```python
from build123d import *

# Parameters (mm, degrees)
SKETCH1_R           = 25.4
BOSS_EXTRUDE1_DEPTH = 33.274
SKETCH2_R           = 22.225
BOSS_EXTRUDE2_DEPTH = 19.05
SKETCH3_R           = 12.7
CUT_EXTRUDE2_DEPTH  = 64.467479673
BOSS_EXTRUDE3_DEPTH = 25.4
FILLET1_R           = 6.35
FILLET2_R           = 6.35
CUT_EXTRUDE3_DEPTH  = 154.088688922
BOSS_EXTRUDE4_DEPTH = 8.128
FILLET3_R           = 6.35


with BuildPart() as part:
    # Sketch1 → Boss-Extrude1 (new body)
    with BuildSketch(Plane.XY):
        Circle(SKETCH1_R)
    extrude(amount=BOSS_EXTRUDE1_DEPTH)

    # Sketch2 → Boss-Extrude2 (add)
    with BuildSketch(Plane.XY.offset(33.274)):
        with Locations(Location((0, 0, 0), (0, 0, 180))):
            Circle(SKETCH2_R)
    extrude(amount=BOSS_EXTRUDE2_DEPTH)

    # Sketch3 → Cut-Extrude2 (cut, through all)
    with BuildSketch(Plane.XY):
        Circle(SKETCH3_R)
    extrude(amount=CUT_EXTRUDE2_DEPTH, mode=Mode.SUBTRACT)

    # Sketch5 → Boss-Extrude3 (add)
    with BuildSketch(Plane(origin=(0, 0, 3.048), x_dir=(-1, 0, 0), z_dir=(0, 0, -1))):
        with BuildLine():
            Line((100.803124952, 12.7), (21.997045256, 12.7))
            ThreePointArc((21.997045256, 12.7), (24.534515988, 6.574003746), (25.4, 0))
            ThreePointArc((25.4, 0), (24.534515988, -6.574003746), (21.997045256, -12.7))
            Line((21.997045256, -12.7), (100.803124952, -12.7))
            ThreePointArc((100.803124952, -12.7), (100.053333913, -17.660418251), (99.059597973, -22.577777778))
            ThreePointArc((99.059597973, -22.577777778), (108.619825498, -37.782449747), (123.824497467, -28.222222222))
            ThreePointArc((123.824497467, -28.222222222), (125.578613792, 18.9476056), (109.985226281, 63.5))
            ThreePointArc((109.985226281, 63.5), (92.636703653, 68.148522628), (87.988181024, 50.8))
            ThreePointArc((87.988181024, 50.8), (96.298711326, 32.390094118), (100.803124952, 12.7))
        make_face()
    extrude(amount=-BOSS_EXTRUDE3_DEPTH)

    # Fillet1
    fillet1_edges = [part.edges().sort_by_distance(p)[0] for p in [
        (-100.803124952, 12.7, 15.748),
    ]]
    fillet(fillet1_edges, radius=FILLET1_R)

    # Fillet2
    fillet2_edges = [part.edges().sort_by_distance(p)[0] for p in [
        (-100.803124952, -12.7, 15.748),
    ]]
    fillet(fillet2_edges, radius=FILLET2_R)

    # Sketch6 → Cut-Extrude3 (cut, through all)
    with BuildSketch(Plane(origin=(0, 0, 3.048), x_dir=(-1, 0, 0), z_dir=(0, 0, -1))):
        with BuildLine():
            Line((44.45, -5.588), (82.55, -5.588))
            ThreePointArc((82.55, -5.588), (88.138, 0), (82.55, 5.588))
            Line((82.55, 5.588), (44.45, 5.588))
            ThreePointArc((44.45, 5.588), (38.862, 0), (44.45, -5.588))
        make_face()
        with BuildLine():
            ThreePointArc((117.620316517, -26.867892407), (119.3040242, 17.971430377), (104.485964967, 60.325))
            ThreePointArc((104.485964967, 60.325), (95.811703653, 62.649261314), (93.487442339, 53.975))
            ThreePointArc((93.487442339, 53.975), (106.745705863, 16.079700863), (105.239230568, -24.039693207))
            ThreePointArc((105.239230568, -24.039693207), (110.015673942, -31.644335781), (117.620316517, -26.867892407))
        make_face()
    extrude(amount=-CUT_EXTRUDE3_DEPTH, mode=Mode.SUBTRACT)

    # Sketch7 → Boss-Extrude4 (add)
    with BuildSketch(Plane.XY.offset(8.128)):
        with BuildLine():
            Line((-93.3255592, 12.7), (-21.997045256, 12.7))
            ThreePointArc((-21.997045256, 12.7), (-10.533208363, 23.11301628), (4.846548483, 24.93333046))
            Line((4.846548483, 24.93333046), (-91.719825153, 43.703932019))
            ThreePointArc((-91.719825153, 43.703932019), (-96.345611399, 32.250320373), (-99.547263147, 20.32))
            ThreePointArc((-99.547263147, 20.32), (-98.24424805, 15.033907372), (-93.3255592, 12.7))
        make_face()
    extrude(amount=BOSS_EXTRUDE4_DEPTH)

    # Fillet3
    # the kernel refuses this fillet: 6.35 mm, written as the material it adds along each edge
    with BuildSketch(Plane(origin=(-91.719825153, 43.703932019, 8.128), x_dir=(0.4664648604868203, 0.8845397299901295, 0), z_dir=(0, 0, 1))) as fillet3_piece_1:
        with BuildLine():
            CenterArc((8.551066202, -6.349980485), FILLET3_R, 90.142046539, 106.663020028)
            Line((2.472249714, -8.185869942), (1.864368065, -8.369458888))
            Line((1.864368065, -8.369458888), (-0.607881649, -0.183588946))
            Line((-0.607881649, -0.183588946), (-0.02578882, 0.634476112))
            ThreePointArc((-0.02578882, 0.634476112), (8.041755062, 0.643812976), (8.533749149, 0.634998049))
            Line((8.533749149, 0.634998049), (8.535323427, 0))
        make_face()
    extrude(amount=8.128)


solid = part.part
```
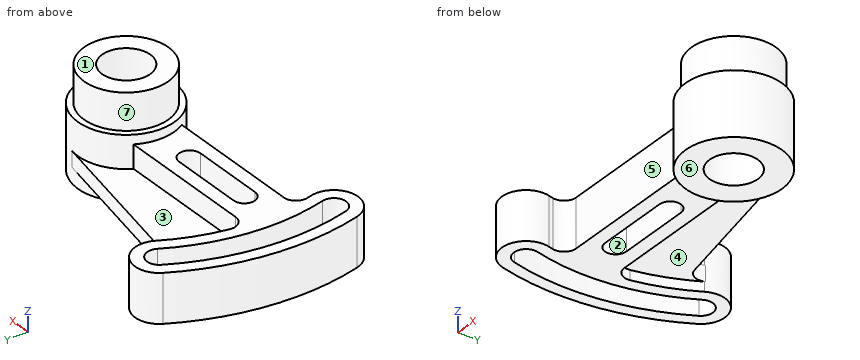
The model under review builds one solid part; all positions refer to its coordinate system, in mm. Face numbers are marked on the shaded views. A direction names the side the tool comes from. Give positions to 0.01 mm unless a question says otherwise; leave off trailing zeros. Order: outer loops, then holes, each group sorted by start corner. A loop starts at its lowest first (then second) coordinate and runs counter-clockwise, first axis right, second up. Notation, with made-up numbers: (-8.75, 4.25) - (25.25, 4.25) arc R22 ccw to (25.25, 28.25) - close; hole circle Ø1 at (77, 3). An arc over 180 degrees is marked (long way). Use CSV: the item, a comma, the result in double quotes. Start each with the question number.
Q1. We need section A-A, the plane y = 0. Write out the cut boundary in (x, z) (3 decimals), and give its area (3 significant figures).
Q2. To check wall thickness, follow line 1 along Y through (x, z) = (0, 26.5); line 2 along X through (y, z) = (0, 26); line 3 along Y through (x, z) = (0, 40.5) (3 decimals). State the ranges of each line that lie inside material, in increasing order. Write a range as [from, to].
Q3. We need section D-D, the plane z = 5. State how many separate pieces and enclosed holes the cut face has, and give its area (3 significant figures).
Q4. Clearance check with flat-ended pins moving along their axes: pin 1 Ø1 at (y, z) = (26.5, 12.5) entering from -X; pin 2 Ø1 at (x, z) = (-86, 24.5) entering from -Y; pin 3 Ø1.5 at (x, z) = (-47, 5) entering from +Y. State where each tip first meets the part, or that it passes through.
Q5. The part is to be moulded in two halves that separate along Y. For the marked faces 4, 5, 6 and 7, say which applies: +Y half, -Y half, draft (parallel to the pull), parting line (faces both ways), or undercut.
Q6. We need section B-B, the plane x = -73.5. Write out the cut boundary in (y, z), and give its area (3 significant figures).
Q7. We need section C-C, the plane y = 57.15. Write out the cut boundary in (x, z), and give its area (3 significant figures).
Q8. Tool access review of the marked faces 1, 2 and 3: name each direction out of +Z, -Z, +X, -X, +Y, -Y from which nothing blocks a thin tool from reaching the whole face with its end or side.
Outcome:
1,outline,"(-127, 3.048) - (-120.65, 3.048) - (-120.65, 28.448) - (-127, 28.448) - close; (-107.95, 3.048) - (-88.138, 3.048) - (-88.138, 28.448) - (-107.95, 28.448) - close; (-38.862, 3.048) - (-25.4, 3.048) - (-25.4, 0) - (-12.7, 0) - (-12.7, 52.324) - (-22.225, 52.324) - (-22.225, 33.274) - (-25.4, 33.274) - (-25.4, 28.448) - (-38.862, 28.448) - close; (12.7, 0) - (25.4, 0) - (25.4, 33.274) - (22.225, 33.274) - (22.225, 52.324) - (12.7, 52.324) - close"
1,area,"2,210 mm^2"
2,line 1,"y = [-25.4, -12.7], [12.7, 25.4]"
2,line 2,"x = [-127, -120.65], [-107.95, -88.14], [-38.86, -12.7], [12.7, 25.4]"
2,line 3,"y = [-22.225, -12.7], [12.7, 22.225]"
3,separate pieces,"1"
3,enclosed holes,"3"
3,area,"4,440 mm^2"
4,pin 1,"stops at x = -124.31"
4,pin 2,"stops at y = -12.7"
4,pin 3,"stops at y = 12.7"
5,face 4,"undercut"
5,face 5,"-Y half"
5,face 6,"draft"
5,face 7,"parting line"
6,outline,"(-12.7, 3.05) - (-5.59, 3.05) - (-5.59, 28.45) - (-12.7, 28.45) - close; (5.59, 3.05) - (12.7, 3.05) - (12.7, 8.13) - (40.16, 8.13) - (40.16, 16.26) - (12.7, 16.26) - (12.7, 28.45) - (5.59, 28.45) - close"
6,area,"585 mm^2"
7,outline,"(-113.41, 3.05) - (-106.26, 3.05) - (-106.26, 28.45) - (-113.41, 28.45) - close; (-92.64, 3.05) - (-86.29, 3.05) - (-86.29, 28.45) - (-92.64, 28.45) - close"
7,area,"343 mm^2"
8,face 1,"+Z, +X, -X, +Y, -Y"
8,face 2,"+Z, -Z"
8,face 3,"+Z"
